Design review of the part built by this model. Coordinates are the model's own, in mm. A direction names the side the tool comes from. Coordinates: 2 decimals unless noted, no trailing zeros. Order: outer loops, then holes, each group sorted by start corner. A loop starts at its lowest first (then second) coordinate and runs counter-clockwise, first axis right, second up. Notation, with made-up numbers: M -23,22 L 7,22 A15 ccw 7,38 Z; hole C 11,66.25 d4. An arc over 180 degrees is marked long. Answer in a Markdown table with one row per item.
from build123d import *

# Parameters (mm, degrees)
F0_R     = 65
F1_DEPTH = 40
F2_DEPTH = 6
F3_DEPTH = 40
F4_R     = 4.7625
F5_DEPTH = 6


with BuildPart() as f1:
    # F0 (on Top) → F1 (new body)
    with BuildSketch(Plane.XY):
        with BuildLine():
            ThreePointArc((63.245553, -30), (68.290514, -15.375488), (70, 0))
            ThreePointArc((70, 0), (68.290514, 15.375488), (63.245553, 30))
            ThreePointArc((63.245553, 30), (-70, 0), (63.245553, -30))
        make_face()
        Circle(F0_R, mode=Mode.SUBTRACT)
    extrude(amount=F1_DEPTH)

    # F0 (on Top) → F2 (join)
    with BuildSketch(Plane.XY):
        with BuildLine():
            ThreePointArc((63.245553, 30), (68.290514, 15.375488), (70, 0))
            ThreePointArc((70, 0), (68.290514, -15.375488), (63.245553, -30))
            Line((63.245553, -30), (104, -30))
            Line((104, -30), (104, 30))
            Line((104, 30), (63.245553, 30))
        make_face()
    extrude(amount=F2_DEPTH)

    # F0 (on Top) → F3 (join)
    with BuildSketch(Plane.XY):
        Polygon((110, 30), (104, 30), (104, -30), (110, -30), (110, 0), align=None)
    extrude(amount=F3_DEPTH)

    # F4 (on face) → F5 (cut)
    with BuildSketch(Plane.YZ.offset(110)):
        with Locations((-15, 23)):
            Circle(F4_R)
        with Locations((15, 23)):
            Circle(F4_R)
    extrude(amount=-F5_DEPTH, mode=Mode.SUBTRACT)


solid = f1.part
(1) Draft analysis for pull direction Z (two halves, no side actions). For faces 1 (the cylindrical face through (107.04, -16.03, 18.35)), 2 (the flat face through (83, 0, 6)), 3 (the cylindrical face through (62, 19.52, 19.72)), state which applies: pulls with the +Z half, pulls with the -Z half, needs draft (parallel to the pull), parting line crosses it, or undercut.
Return value:
| item | result |
|---|---|
| face 1 | undercut |
| face 2 | pulls with the +Z half |
| face 3 | needs draft |
(2) Insertion check: pin 1 Ø5 at (x, y) = (82.5, -13) entering from +Z; pin 2 Ø5 at (x, z) = (56.5, 12) entering from +Y; pin 3 Ø10 at (y, z) = (-53, 28.5) entering from +X. Each pin has a flat end and moves straight along its axis. Give the tip position at first contact, or say it passes through.
Return value:
| item | result |
|---|---|
| pin 1 | stops at z = 6 |
| pin 2 | stops at y = 44.54 |
| pin 3 | stops at x = 50.95 |
(3) Add section B-B, the plane x = 0. Give the boundary of the cut face in (y, z).
Return value:
| item | result |
|---|---|
| outline | M -70,0 L -65,0 L -65,40 L -70,40 Z; M 65,0 L 70,0 L 70,40 L 65,40 Z |
(4) For faces 4 (the flat face through (104, 0, 23)), 5 (the flat face through (66, 6, 0)), 6 (the cylindrical face through (107.04, 13.97, 18.35)), 7 (the flat face through (97, 30, 5)), 8 (the flat face through (95, -30, 4)), list the 3-axis set-ups (+Z, -Z, +X, -X, +Y, -Y) from which the entire face can be reached by the end or side of a thin tool; tool diameter is ignored.
Return value:
| item | result |
|---|---|
| face 4 | +Z, +Y, -Y |
| face 5 | -Z, +X, -X, +Y, -Y |
| face 6 | +X |
| face 7 | +Z, -Z, +X, +Y |
| face 8 | +Z, -Z, +X, -Y |
(5) Add section A-A, the plane z = 23. Give the boundary of the cut face in (x, y).
Return value:
| item | result |
|---|---|
| outline | M 63.25,-30 A70 ccw 70,0 A70 ccw 63.25,30 A70 ccw long Z; M 104,-30 L 110,-30 L 110,-19.76 L 104,-19.76 Z; M 104,-10.24 L 110,-10.24 L 110,10.24 L 104,10.24 Z; M 104,19.76 L 110,19.76 L 110,30 L 104,30 Z; hole C 0,0 d130 |
(6) Add section D-D, the plane y = -15. Give the boundary of the cut face in (x, z).
Return value:
| item | result |
|---|---|
| outline | M -68.37,0 L -63.25,0 L -63.25,40 L -68.37,40 Z; M 63.25,0 L 110,0 L 110,18.24 L 104,18.24 L 104,6 L 68.37,6 L 68.37,40 L 63.25,40 Z; M 104,27.76 L 110,27.76 L 110,40 L 104,40 Z |
(7) Add section C-C, the plane y = 55. Give the boundary of the cut face in (x, z).
Return value:
| item | result |
|---|---|
| outline | M -43.3,0 L -34.64,0 L -34.64,40 L -43.3,40 Z; M 34.64,0 L 43.3,0 L 43.3,40 L 34.64,40 Z |
(8) For line 1 along X through (y, z) = (1, 20); line 2 along Z through (x, y) = (105, 15); line 3 along X through (y, z) = (17, 36), list the stretches that pass through material, from the lowest coordinate up. Write a range as from..to.
Return value:
| item | result |
|---|---|
| line 1 | x = -69.99..-64.99, 64.99..69.99, 104..110 |
| line 2 | z = 0..18.24, 27.76..40 |
| line 3 | x = -67.9..-62.74, 62.74..67.9, 104..110 |
